Source: CAD feature listing. Evaluate the final solid. Frame: model axes, mm. Face numbers are marked on the shaded views. A direction names the side the tool comes from. Give positions to 0.01 mm unless a question says otherwise; leave off trailing zeros. Loops run counter-clockwise (first coordinate to the right, second up) from the corner with the lowest first, then second, coordinate; pieces in that order, holes last.
Autodesk Inventor part; units mm, degrees
ref_plane "YZ Plane" through (0, 0, 0) normal (1, 0, 0) x (0, 1, 0)
ref_plane "XZ Plane" through (0, 0, 0) normal (0, 1, 0) x (-1, 0, 0)
ref_plane "XY Plane" through (0, 0, 0) normal (0, 0, 1) x (1, 0, 0)
sketch "Sketch1" plane through (0, 0, 0) normal (0, 0, 1) x (1, 0, 0)
  circle A0 centre (0, 0) radius 25.4
  dimension "d0" = 50.8
extrude "Extrusion1" add sketch "Sketch1" along normal blind 6.35
sketch "Sketch2" plane through (0, 0, 6.35) normal (0, 0, 1) x (1, 0, 0)
  circle A0 centre (0, 0) radius 6.35
  dimension "d3" = 12.7
extrude "Extrusion2" add sketch "Sketch2" along normal blind 57.15
sketch "Sketch3" plane through (0, 0, 0) normal (0, 0, -1) x (-1, 0, 0)
  circle A0 centre (0, 0) radius 6.35
  circle A1 centre (0, 0) radius 9.525
  dimension "d6" = 19.05
extrude "Extrusion3" add sketch "Sketch3" along normal blind 19.05
sketch "Sketch4" plane through (0, 0, -19.05) normal (0, 0, -1) x (-1, 0, 0)
  circle A0 centre (0, 0) radius 9.525
  circle A1 centre (0, 0) radius 9.525 construction
  line L0 (-9.525, 0) -> (9.525, 0) construction
  line L1 (-9.525, 0) -> (9.525, 0)
  line L2 (9.525, 0) -> (9.525, -93.9249)
  line L3 (9.525, -93.9249) -> (-9.525, -93.9249)
  line L4 (-9.525, -93.9249) -> (-9.525, 0)
  dimension "d9" = 19.05
  dimension "d10" = 93.9249
extrude "Extrusion4" add sketch "Sketch4" against normal blind 19.05 contours L2 L3 L4 A0
extrude "Extrusion6" add sketch "Sketch3" along normal blind 19.05 contours A0
equation "\"d0\" = OG_gearDiameter"
equation "\"d1\" = OG_gearThickness"
equation "\"d3\" = OG_shaftDiameter"
equation "\"d4\" = OG_shaftLength"
equation "\"d6\" = LE_baseDiameter"
equation "\"d7\" = LE_thickness"
equation "\"d9\" = LE_thickness"
equation "\"d10\" = LE_maxLength"
equation "\"d11\" = LE_thickness"
equation "\"d15\" = LE_thickness + LE_offsetAboveOuterGear"
equation "\"Wheel_Related_W_\" = 0"
equation "\"W_innerDiameter\" = 254"
equation "\"W_innerDepth\" = 50.8"
equation "\"W_wallThickness\" = 6.35"
equation "\"W_holesClearance\" = 0.254"
equation "\"W_outerGearHoleDiameter\" = 13.208"
equation "\"W_innerGearHoleDiameter\" = 38.608"
equation "\"TempSpotReserved7\" = 0"
equation "\"TempSpotReserved8\" = 0"
equation "\"TempSpotReserved9\" = 0"
equation "\"TempSpotReserved10\" = 0"
equation "\"TempSpotReserved11\" = 0"
equation "\"TempSpotReserved12\" = 0"
equation "\"TempSpotReserved13\" = 0"
equation "\"TempSpotReserved14\" = 0"
equation "\"TempSpotReserved15\" = 0"
equation "\"TempSpotReserved16\" = 0"
equation "\"TempSpotReserved17\" = 0"
equation "\"TempSpotReserved18\" = 0"
equation "\"TempSpotReserved19\" = 0"
equation "\"TempSpotReserved20\" = 0"
equation "\"Inner_Gear_Related_IG_\" = 0"
equation "\"IG_shaftDiameter\" = 25.4"
equation "\"IG_gearDiameter\" = 127"
equation "\"IG_shaftLength\" = 127"
equation "\"IG_gearThickness\" = 6.35"
equation "\"TempSpotReserved25\" = 0"
equation "\"TempSpotReserved26\" = 0"
equation "\"TempSpotReserved27\" = 0"
equation "\"TempSpotReserved28\" = 0"
equation "\"TempSpotReserved29\" = 0"
equation "\"TempSpotReserved30\" = 0"
equation "\"TempSpotReserved31\" = 0"
equation "\"TempSpotReserved32\" = 0"
equation "\"TempSpotReserved33\" = 0"
equation "\"TempSpotReserved34\" = 0"
equation "\"TempSpotReserved35\" = 0"
equation "\"TempSpotReserved36\" = 0"
equation "\"TempSpotReserved37\" = 0"
equation "\"TempSpotReserved38\" = 0"
equation "\"TempSpotReserved39\" = 0"
equation "\"TempSpotReserved40\" = 0"
equation "\"Outer_Gear_Related_OG_\" = 0"
equation "\"OG_distanceFromCenter\" = 88.9"
equation "\"OG_shaftDiameter\" = 12.7"
equation "\"OG_gearDiameter\" = 50.8"
equation "\"OG_shaftLength\" = 57.15"
equation "\"OG_gearThickness\" = 6.35"
equation "\"TempSpotReserved47\" = 0"
equation "\"TempSpotReserved48\" = 0"
equation "\"TempSpotReserved49\" = 0"
equation "\"TempSpotReserved50\" = 0"
equation "\"TempSpotReserved51\" = 0"
equation "\"TempSpotReserved52\" = 0"
equation "\"TempSpotReserved53\" = 0"
equation "\"TempSpotReserved54\" = 0"
equation "\"TempSpotReserved55\" = 0"
equation "\"TempSpotReserved56\" = 0"
equation "\"TempSpotReserved57\" = 0"
equation "\"TempSpotReserved58\" = 0"
equation "\"TempSpotReserved59\" = 0"
equation "\"TempSpotReserved60\" = 0"
equation "\"Leg_Extensions_Related_LE_\" = 0"
equation "\"LE_baseDiameter\" = 19.05"
equation "\"LE_maxLength\" = 93.92488"
equation "\"LE_thickness\" = 19.05"
equation "\"IG_ratioToOuterGear\" = 2.5"
equation "\"B_bearingThickness\" = 6.35"
equation "\"TempSpotReserved43\" = 0"
equation "\"TempSpotReserved45\" = 0"
equation "\"Thisisatest\" = 25.4"
equation "\"TempSpotReserved46\" = 0"
equation "\"TempSpotReserved44\" = 0"
equation "\"LE_offsetAboveOuterGear\" = 0"
equation "\"Bearing_Related_B_\" = 0"
equation "\"TempSpotReserved42\" = 0"
properties part number "outerGear_2"
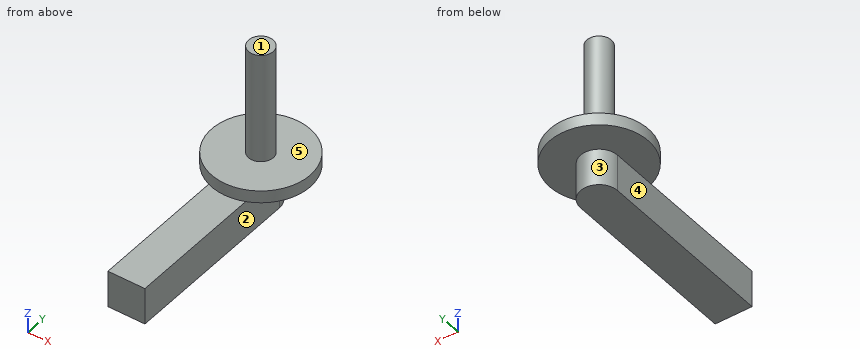
(1) Section A-A, the plane x = 0. Return the cut outline in (y, z) (3 decimals).
A:
outline: (-93.925, -19.05) - (9.525, -19.05) - (9.525, 0) - (25.4, 0) - (25.4, 6.35) - (6.35, 6.35) - (6.35, 63.5) - (-6.35, 63.5) - (-6.35, 6.35) - (-25.4, 6.35) - (-25.4, 0) - (-93.925, 0) - close
(2) First-contact query: pin 1 (10 mm diameter, centred on y = -50.5, z = -9.5, fed in from +X) (3 decimals); pin 2 (15 mm diameter, centred on y = -36.5, z = -8.5, fed in from -X) (3 decimals); pin 3 (15 mm diameter, centred on x = 3, y = -72, fed in from +Z); pin 4 (24.5 mm diameter, centred on x = 10, y = 9.5, fed in from -Z). Flat tips, straight axial feed; report the tip coordinate or a pass-through.
A:
pin 1: stops at x = 9.525
pin 2: stops at x = -9.525
pin 3: stops at z = 0
pin 4: stops at z = -19.05
(3) Section B-B, the plane z = 22. Return the cut outline in (x, y), then the cut area to 3 significant figures.
A:
outline: circle Ø12.7 at (0, 0)
area: 127 mm2
(4) Section C-C, the plane y = -33. Return the cut outline in (x, z) (3 decimals).
A:
outline: (-9.525, -19.05) - (9.525, -19.05) - (9.525, 0) - (-9.525, 0) - close
(5) Section D-D, the plane z = 2. Return the cut outline in (x, y), then the cut area to 3 significant figures.
A:
outline: circle Ø50.8 at (0, 0)
area: 2,030 mm2
(6) Ray query, line 1 along X through (y, z) = (-46.5, -1) (3 decimals); line 2 along Z through (x, y) = (20.5, 13); line 3 along Z through (x, y) = (-7.5, -45.5). Return the intervals inside material, ascending.
A:
line 1: x = -9.525 to 9.525
line 2: z = 0 to 6.35
line 3: z = -19.05 to 0
(7) Reachability of the marked faces 1, 2, 3, 4 and 5 from +Z, -Z, +X, -X, +Y, -Y: full face, straight path, thin tool, end or side. Return the list, or none.
A:
face 1: +Z, +X, -X, +Y, -Y
face 2: -Z, +X, +Y, -Y
face 3: -Z, +Y
face 4: -Z, -X, +Y, -Y
face 5: +Z
